Build history of the part. All positions in model axes, mm. Round coordinates to 2 decimals unless told otherwise and drop trailing zeros. Write each loop counter-clockwise with the first axis right and the second up, starting at its lowest first coordinate (ties: lowest second). Pieces come first, ordered by that corner, then holes. Notation, with made-up numbers: M -38.5,34.25 L -31.5,34.25 A27 cw -31.5,66.25 Z; hole C 18.25,58 d11. An arc over 180 degrees is marked long. Use a Markdown table: item, result.
from build123d import *

# Parameters (mm, degrees)
F0_W     = 103.187494
F0_H     = 63.5
F1_DEPTH = 76.2
F2_R     = 5.08


with BuildPart() as f1:
    # F0 (on Front) → F1 (new body)
    with BuildSketch(Plane.XZ):
        Rectangle(F0_W, F0_H)
        Polygon((51.593747, -31.75), (-51.593747, -31.75), (0, -57.150003), align=None)
    extrude(amount=F1_DEPTH)

    # F2
    f2_edges = [f1.edges().sort_by_distance(p)[0] for p in [
        (0, -76.2, 31.75),
        (-51.593747, -76.2, 0),
        (-25.796873, -76.2, -44.450001),
        (25.796873, -76.2, -44.450001),
        (51.593747, -76.2, 0),
    ]]
    fillet(f2_edges, radius=F2_R)


solid = f1.part
Q1. Drop flat-ended pins along their axis: P1, Ø3, axis at x = 24.5, z = 4, coming from the +Y side; P2, Ø5, axis at x = 29.5, y = -23, coming from the -Z side. Give the stop position or say it passes through.
Response values:
| item | result |
|---|---|
| P1 | stops at y = 0 |
| P2 | stops at z = -43.86 |
Q2. Cut at A-A on y = -29. Give the cut face in (x, z).
Response values:
| item | result |
|---|---|
| outline | M -51.59,-31.75 L 0,-57.15 L 51.59,-31.75 L 51.59,31.75 L -51.59,31.75 Z |
Q3. Drill centre lines: L1, parallel to Z at x = 27.5, y = -37; L2, parallel to Z at x = -16.5, y = -60; L3, parallel to Y at x = 19, z = -43. Where is each one in solid material? Low to high.
Response values:
| item | result |
|---|---|
| L1 | z = -43.61 to 31.75 |
| L2 | z = -49.03 to 31.75 |
| L3 | y = -76.14 to 0 |
